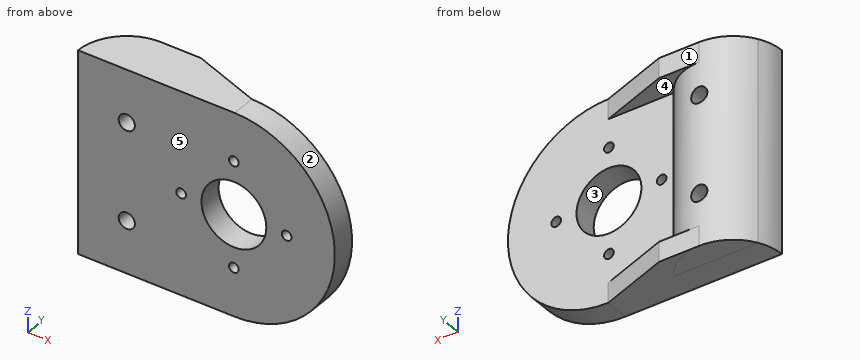
from build123d import *

# Parameters (mm, degrees)
CROQUIS1_R              = 0.599999868
CROQUIS1_R_2            = 3.999426158
CROQUIS1_R_3            = 1.000000121
CROQUIS1_R_4            = 1.000000477
SALIENTE_EXTRUIR1_DEPTH = 3
SALIENTE_EXTRUIR2_DEPTH = 24.89496
CROQUIS3_W              = 13.299999714
CROQUIS3_H              = 2.45
SALIENTE_EXTRUIR3_DEPTH = 3
CORTAR_EXTRUIR1_DEPTH   = 24.89496
CROQUIS5_R              = 1.000000121
CROQUIS5_R_2            = 1.000000477
CORTAR_EXTRUIR2_DEPTH   = 11


with BuildPart() as part:
    # Croquis1 → Saliente-Extruir1 (new body)
    with BuildSketch(Plane(origin=(0, 0, 0), x_dir=(1, 0, 0), z_dir=(0, 1, 0))):
        with BuildLine():
            Line((4.218422555, -12.81969876), (-15.081577159, -12.81969876))
            Line((-15.081577159, -12.81969876), (-15.081577159, 12.075260967))
            Line((-15.081577159, 12.075260967), (4.218422555, 12.075260967))
            ThreePointArc((4.218422555, 12.075260967), (16.567050884, -0.372218896), (4.218422555, -12.81969876))
        make_face()
        with Locations((4.118422395, 6.128403493)):
            Circle(CROQUIS1_R, mode=Mode.SUBTRACT)
        with Locations((4.119175364, -0.372218896)):
            Circle(CROQUIS1_R_2, mode=Mode.SUBTRACT)
        with Locations((-9.081577367, 5.628403394)):
            Circle(CROQUIS1_R_3, mode=Mode.SUBTRACT)
        with Locations((-9.081576585, -6.371596672)):
            Circle(CROQUIS1_R_4, mode=Mode.SUBTRACT)
        with Locations((10.620712828, -0.371667036)):
            Circle(CROQUIS1_R, mode=Mode.SUBTRACT)
        with Locations((4.1206423, -6.873957469)):
            Circle(CROQUIS1_R, mode=Mode.SUBTRACT)
        with Locations((-2.381648134, -0.373886941)):
            Circle(CROQUIS1_R, mode=Mode.SUBTRACT)
    extrude(amount=SALIENTE_EXTRUIR1_DEPTH)

    # Croquis2 → Saliente-Extruir2 (add)
    with BuildSketch(Plane.XY.offset(12.81969876)):
        with BuildLine():
            Line((-14.277729582, 3), (-3.885424736, 3))
            ThreePointArc((-3.885424736, 3), (-9.081577159, 6), (-14.277729582, 3))
        make_face()
    extrude(amount=-SALIENTE_EXTRUIR2_DEPTH)

    # Croquis3 → Saliente-Extruir3 (add)
    with BuildSketch(Plane(origin=(0, 3, 0), x_dir=(1, 0, 0), z_dir=(0, 1, 0))):
        with Locations((-2.431577302, -11.59469876)):
            Rectangle(CROQUIS3_W, CROQUIS3_H)
        with Locations((-2.431577302, 10.850260967)):
            Rectangle(CROQUIS3_W, CROQUIS3_H)
    extrude(amount=SALIENTE_EXTRUIR3_DEPTH)

    # Croquis4 → Cortar-Extruir1 (cut)
    with BuildSketch(Plane.XY.offset(12.81969876)):
        Polygon((-4.171577445, 6), (4.218422555, 3), (4.218422555, 6), align=None)
        with BuildLine():
            Line((-15.081577159, 0), (-16.256016644, 0))
            ThreePointArc((-16.256016644, 0), (-14.36312843, 4.855697487), (-9.683294652, 7.149162047))
            Line((-9.683294652, 7.149162047), (-9.683294652, 5.969751759))
            ThreePointArc((-9.683294652, 5.969751759), (-13.53187518, 4.024282237), (-15.081577159, 0))
        make_face()
    extrude(amount=-CORTAR_EXTRUIR1_DEPTH, mode=Mode.SUBTRACT)

    # Croquis5 → Cortar-Extruir2 (cut)
    with BuildSketch(Plane.XZ):
        with Locations((-9.081577367, -5.628403394)):
            Circle(CROQUIS5_R)
        with Locations((-9.081576585, 6.371596672)):
            Circle(CROQUIS5_R_2)
    extrude(amount=-CORTAR_EXTRUIR2_DEPTH, mode=Mode.SUBTRACT)


solid = part.part
Build history of the part. All positions in model axes, mm. Face numbers are marked on the shaded views. A direction names the side the tool comes from. Round coordinates to 2 decimals unless told otherwise and drop trailing zeros. Order: outer loops, then holes, each group sorted by start corner. A loop starts at its lowest first (then second) coordinate and runs counter-clockwise, first axis right, second up. Notation, with made-up numbers: M -25,81.25 L 3,81.25 A34 ccw 3,116.25 Z; hole C 88.5,53 d2. An arc over 180 degrees is marked long. Use CSV: the item, a comma, the result in double quotes. Start each with the question number.
(1) Cut at B-B on x = -9.5. List the corners of the cut face in (y, z), then the cut area to 3 significant figures.
(2) Tool access for the marked faces 4 and 5: list every direction of +Z, -Z, +X, -X, +Y, -Y with a clear straight run to the whole face (end or side of a thin tool).
(3) Flat gauge pins, fed straight in: P1, Ø10, axis at x = 6.5, z = -4.5, coming from the +Y side; P2, Ø2, axis at x = 1, y = 5.5, coming from the +Z side; P3, Ø12, axis at x = -9, z = 6, coming from the -Y side; P4, Ø2, axis at y = 4.5, z = -1, coming from the +X side. Where does each tip first touch, or does it go through?
(4) Cut at A-A on z = 3. List the corners of the cut face in (x, y), then the cut area to 3 significant figures.
(5) Drill centre lines: probe 1 along Z at (x, y) = (-9, 5); probe 2 along Z at (x, y) = (0, 4); probe 3 along X at (y, z) = (0.5, 3.75). Where is each one in solid material? Low to high.
(6) Mould opens along Z. For the marked faces 1, 2 and 3 say: +Z half, -Z half, draft (parallel to the pull), parting line (faces both ways), or undercut.
(7) Cut at D-D on y = 5. List the corners of the cut face in (x, z), then the cut area to 3 significant figures.
(8) Cut at C-C on y = 2.5. List the corners of the cut face in (x, z), then the cut area to 3 significant figures.
Findings:
1,outline,"M 0,-12.08 L 5.99,-12.08 L 5.99,-6.54 L 0,-6.54 Z; M 0,-4.72 L 5.99,-4.72 L 5.99,5.46 L 0,5.46 Z; M 0,7.28 L 5.99,7.28 L 5.99,12.82 L 0,12.82 Z"
1,area,"127 mm^2"
2,face 4,"+X, +Y"
2,face 5,"+Z, -Z, +X, -X, -Y"
3,P1,"stops at y = 3"
3,P2,"passes through"
3,P3,"stops at y = 0"
3,P4,"stops at x = -4.21"
4,outline,"M -15.08,0 L 1.1,0 L 1.1,3 L -3.89,3 A6 ccw Z; M 7.13,0 L 16.29,0 L 16.29,3 L 7.13,3 Z"
4,area,"97.3 mm^2"
5,probe 1,"z = -12.08 to -6.63, -4.63 to 5.37, 7.37 to 12.82"
5,probe 2,"z = -12.08 to -9.63, 10.37 to 12.82"
5,probe 3,"x = -15.06 to 1.98, 6.26 to 16.1"
6,face 1,"draft"
6,face 2,"parting line"
6,face 3,"undercut"
7,outline,"M -12.4,-12.08 L -1.37,-12.08 L -1.37,-9.63 L -5.76,-9.63 L -5.76,10.37 L -1.37,10.37 L -1.37,12.82 L -12.4,12.82 Z; hole C -9.08,-5.63 d2; hole C -9.08,6.37 d2"
7,area,"180 mm^2"
8,outline,"M -14.54,-12.08 L 4.22,-12.08 A12.45 ccw 4.22,12.82 L -14.54,12.82 Z; hole C -9.08,-5.63 d2; hole C -9.08,6.37 d2; hole C -2.38,0.37 d1.2; hole C 4.12,0.37 d8; hole C 4.12,-6.13 d1.2; hole C 4.12,6.87 d1.2; hole C 10.62,0.37 d1.2"
8,area,"647 mm^2"
